Read the model definition and answer for the solid it produces. Units are mm, in the model's axes. Coordinates: 2 decimals unless noted, no trailing zeros. Loops run counter-clockwise (first coordinate to the right, second up) from the corner with the lowest first, then second, coordinate; pieces in that order, holes last.
from build123d import *

# Parameters (mm, degrees)
F0_R     = 33.02
F0_R_2   = 3.175
F1_DEPTH = 5.08
F2_R     = 33.02
F2_R_2   = 30.48
F3_DEPTH = 25.4
F5_DEPTH = 5.08


with BuildPart() as f1:
    # F0 (on Top) → F1 (new body)
    with BuildSketch(Plane.XY):
        Circle(F0_R)
        Circle(F0_R_2, mode=Mode.SUBTRACT)
    extrude(amount=F1_DEPTH)

    # F2 (on face) → F3 (join)
    with BuildSketch(Plane.XY.offset(5.08)):
        Circle(F2_R)
        Circle(F2_R_2, mode=Mode.SUBTRACT)
    extrude(amount=F3_DEPTH)

    # F4 (on face) → F5 (join)
    with BuildSketch(Plane(origin=(0, 0, 0), x_dir=(1, 0, 0), z_dir=(0, 0, -1))):
        with BuildLine():
            Line((0, 29.845), (0, 26.035))
            ThreePointArc((0, 26.035), (1.347038, 26.592962), (1.905, 27.94))
            ThreePointArc((1.905, 27.94), (1.347038, 29.287038), (0, 29.845))
        make_face()
        with BuildLine():
            ThreePointArc((0, 29.845), (-1.905, 27.94), (0, 26.035))
            Line((0, 26.035), (0, 29.845))
        make_face()
    extrude(amount=F5_DEPTH)


solid = f1.part
Item 1: A cutting plane is placed at D-D on z = 16.5. Determine the outline of the cut face in (x, y), then the cut area to 3 significant figures.
Numbers:
outline: circle Ø66.04 at (0, 0); hole circle Ø60.96 at (0, 0)
area: 507 mm2
Item 2: Find the intervals of material crossed by line 1 along X through (y, z) = (-1, 20); line 2 along Z through (x, y) = (-9.5, 16); line 3 along X through (y, z) = (2.5, 26.5), in increasing order.
Numbers:
line 1: x = -33 to -30.46, 30.46 to 33
line 2: z = 0 to 5.08
line 3: x = -32.93 to -30.38, 30.38 to 32.93
Item 3: A cutting plane is placed at B-B on x = 26.5. Determine the outline of the cut face in (y, z).
Numbers:
outline: (-19.7, 0) - (19.7, 0) - (19.7, 30.48) - (15.06, 30.48) - (15.06, 5.08) - (-15.06, 5.08) - (-15.06, 30.48) - (-19.7, 30.48) - close
Item 4: A cutting plane is placed at A-A on y = 0. Determine the outline of the cut face in (x, z) (3 decimals), then the cut area to 3 significant figures.
Numbers:
outline: (-33.02, 0) - (-3.175, 0) - (-3.175, 5.08) - (-30.48, 5.08) - (-30.48, 30.48) - (-33.02, 30.48) - close; (3.175, 0) - (33.02, 0) - (33.02, 30.48) - (30.48, 30.48) - (30.48, 5.08) - (3.175, 5.08) - close
area: 432 mm2
Item 5: A cutting plane is placed at C-C on y = -13. Determine the outline of the cut face in (x, z).
Numbers:
outline: (-30.35, 0) - (30.35, 0) - (30.35, 30.48) - (27.57, 30.48) - (27.57, 5.08) - (-27.57, 5.08) - (-27.57, 30.48) - (-30.35, 30.48) - close
Item 6: Determine the mould class of faces 1 (the face through (31.5, 9.9, 15)), 2 (the face through (6, 0, 5.08)), 3 (the face through (0, -28, -5.08)), 4 (the face through (-6.607, -29.755, 17.602)) for opening direction Y: released by +Y, released by -Y, zero draft, split by the parting line, or undercut.
Numbers:
face 1: split by the parting line
face 2: undercut
face 3: zero draft
face 4: undercut
Item 7: Given pin 1 (6 mm diameter, centred on y = 22.5, z = -1.5, fed in from -X); pin 2 (10 mm diameter, centred on x = 19, z = 12, fed in from -Y); pin 3 (6 mm diameter, centred on x = -6.5, y = -26, fed in from +Z); pin 4 (6 mm diameter, centred on y = -1, z = 17, fed in from -X), each flat-ended and moving along its own axis, determine where each tip first touches the part or whether it passes through.
Numbers:
pin 1: stops at x = -26.35
pin 2: stops at y = -29.91
pin 3: stops at z = 5.08
pin 4: stops at x = -33.02
